The listing builds one solid part. Answer for the finished solid, in the listing's coordinates (mm). Face numbers are marked on the shaded views. A direction names the side the tool comes from. Round coordinates to 2 decimals unless told otherwise and drop trailing zeros. Write each loop counter-clockwise with the first axis right and the second up, starting at its lowest first coordinate (ties: lowest second). Pieces come first, ordered by that corner, then holes. Notation, with made-up numbers: (54.5, -29.5) - (108.5, -29.5) arc R11 cw to (108.5, -21.5) - close; hole circle Ø7 at (-7.75, 4). An arc over 180 degrees is marked (long way). Answer as CSV lines item,"result". Start each with the question number.
Item 1: Straight lines are drawn through the part: line 1 along Z through (x, y) = (9.5, 86); line 2 along Y through (x, z) = (40.5, -60.5); line 3 along Y through (x, z) = (65.5, 11). For each, find the intervals that lie inside material, in ascending order. Write a range as [from, to].
Item 2: Flat-ended cylindrical pins translate along their axes: pin 1 (4 mm diameter, centred on x = 48, y = 37, fed in from -Z); pin 2 (3 mm diameter, centred on y = -17, z = -73.5, fed in from +X); pin 3 (3 mm diameter, centred on x = 21, z = -42.5, fed in from +Y); pin 4 (6 mm diameter, centred on x = 50, y = 12.5, fed in from -Z). Find the tip coordinate at first contact, or state that the pin passes through.
Item 3: A cutting plane is placed at A-A on y = 5. Determine the outline of the cut face in (x, z).
Item 4: For a pull along Y with two mould halves and no side action, classify the marked faces 4, 5, 6 and 7 as pulls with the +Y half, pulls with the -Y half, needs draft (parallel to the pull), parting line crosses it, or undercut.
Item 5: Which of the six approach directions +Z, -Z, +X, -X, +Y, -Y give full straight-line access (tool end or side, diameter ignored) to the marked faces 1, 2 and 3?
```python
from build123d import *
from OCP.BRepFilletAPI import BRepFilletAPI_MakeChamfer

# Parameters (mm, degrees)
BOSS_EXTRUDE1_DEPTH = 90
CUT_EXTRUDE1_DEPTH  = 165.439594476
SKETCH4_R           = 37.5
CUT_EXTRUDE2_DEPTH  = 20
CUT_EXTRUDE2_DRAFT  = -6.81
SKETCH5_R           = 8
CUT_EXTRUDE3_DEPTH  = 160.138304628
SKETCH6_R           = 10
CUT_EXTRUDE4_DEPTH  = 2
FILLET1_R           = 45
CUT_EXTRUDE5_DEPTH  = 160.138304628
CHAMFER1_SIZE       = 3
CHAMFER2_SIZE       = 1
CHAMFER2_SIZE2      = 1.14368379
FILLET3_R           = 2
SKETCH8_R           = 2
CUT_EXTRUDE6_DEPTH  = 173.409396496


with BuildPart() as part:
    # Sketch1 → Boss-Extrude1 (new body)
    with BuildSketch(Plane(origin=(0, 0, 0), x_dir=(0, 0, -1), z_dir=(1, 0, 0))):
        Polygon((0, 0), (85, 0), (85, -30), (-25.553583916, -30), (-25.553583916, 100), (-9.553583916, 100), (-9.553583916, 80), align=None)
    extrude(amount=BOSS_EXTRUDE1_DEPTH)

    # Sketch2 → Cut-Extrude1 (cut, through all)
    with BuildSketch(Plane(origin=(0, 0, 9.553583916), x_dir=(-1, 0, 0), z_dir=(0, 0, -1))):
        with BuildLine():
            Line((-70.5, 95), (-70.5, 85))
            ThreePointArc((-70.5, 85), (-72.75, 82.75), (-75, 85))
            Line((-75, 85), (-75, 95))
            ThreePointArc((-75, 95), (-72.75, 97.25), (-70.5, 95))
        make_face()
        with BuildLine():
            Line((-19.5, 95), (-19.5, 85))
            ThreePointArc((-19.5, 85), (-17.25, 82.75), (-15, 85))
            Line((-15, 85), (-15, 95))
            ThreePointArc((-15, 95), (-17.25, 97.25), (-19.5, 95))
        make_face()
    extrude(amount=-CUT_EXTRUDE1_DEPTH, mode=Mode.SUBTRACT)


with BuildPart() as cut_extrude2_tool:
    # Sketch4 → Cut-Extrude2 (with draft: the straight prism first)
    with BuildSketch(Plane(origin=(0, 0, 0), x_dir=(1, 0, 0), z_dir=(0, 1, 0))):
        with Locations((45, 42.5)):
            Circle(SKETCH4_R)
    extrude(amount=-CUT_EXTRUDE2_DEPTH)
    # Cut-Extrude2: the draft: its side faces are tilted about the plane it starts from
    cut_extrude2_sides = [cut_extrude2_tool.faces().sort_by_distance(p)[0] for p in [
        (7.5, -10, -42.5),
    ]]
    draft(cut_extrude2_sides, Plane(origin=(0, 0, 0), x_dir=(1, 0, 0), z_dir=(0, 1, 0)), CUT_EXTRUDE2_DRAFT)


with BuildPart() as part_1:
    add(part.part)

    # Cut-Extrude2: cut by cut_extrude2_tool
    add(cut_extrude2_tool.part, mode=Mode.SUBTRACT)

    # Sketch5 → Cut-Extrude3 (cut, through all)
    with BuildSketch(Plane(origin=(0, 0, 0), x_dir=(-1, 0, 0), z_dir=(0, 0.11857727167698189, -0.9929448275919681))):
        with Locations(Location((-45, 55.568424123, 0), (0, 0, 90))):
            Circle(SKETCH5_R)
    extrude(amount=-CUT_EXTRUDE3_DEPTH, mode=Mode.SUBTRACT)

    # Sketch6 → Cut-Extrude4 (cut)
    with BuildSketch(Plane(origin=(0, 0, 0), x_dir=(-1, 0, 0), z_dir=(0, 0.11857727167698189, -0.9929448275919681))):
        with Locations(Location((-45, 55.568424123, 0), (0, 0, 90))):
            Circle(SKETCH6_R)
    extrude(amount=-CUT_EXTRUDE4_DEPTH, mode=Mode.SUBTRACT)

    # Fillet1
    fillet1_edges = [part_1.edges().sort_by_distance(p)[0] for p in [
        (0, -15, -85),
        (90, -15, -85),
    ]]
    fillet(fillet1_edges, radius=FILLET1_R - 0.0001)  # a hair under: the kernel refuses the full size

    # Sketch7 → Cut-Extrude5 (cut, through all)
    with BuildSketch(Plane(origin=(0, 0, 0), x_dir=(-1, 0, 0), z_dir=(0, 0.11857727167698176, -0.9929448275919681))):
        Polygon((-45, 32.853259254), (-66.213203436, 11.640055819), (-23.786796564, 11.640055819), align=None)
        Polygon((-80.494028285, 18.572434405), (-59.280824849, 39.78563784), (-80.494028285, 60.998841276), align=None)
        Polygon((-30.719175151, 39.78563784), (-9.505971715, 60.998841276), (-9.505971715, 18.572434405), align=None)
    extrude(amount=-CUT_EXTRUDE5_DEPTH, mode=Mode.SUBTRACT)

    # Chamfer1
    chamfer1_edges = [part_1.edges().sort_by_distance(p)[0] for p in [
        (34.393398282, 22.089703532, 2.637947955),
        (55.606601718, 22.089703532, 2.637947955),
        (45, 11.557933218, 1.380246061),
        (20.112573433, 28.973172992, 3.459970494),
        (9.505971715, 39.504943306, 4.717672387),
        (20.112573433, 50.03671362, 5.97537428),
        (80.494028285, 39.504943306, 4.717672387),
        (69.887426567, 28.973172992, 3.459970494),
        (69.887426567, 50.03671362, 5.97537428),
    ]]
    chamfer(chamfer1_edges, length=CHAMFER1_SIZE)

    # Chamfer2: one chamfer whose edges measure the first distance from different faces: ONE call of the kernel's chamfer builder (chamfer() names one face for all edges)
    chamfer2_edges_1 = [part_1.edges().sort_by_distance(p)[0] for p in [
        (9.888395979, -20, -42.5),
    ]]
    chamfer2_side_1 = [part_1.faces().sort_by_distance(p)[0] for p in [
        (8.694197989, -10, -42.5),
    ]]
    chamfer2_edges_2 = [part_1.edges().sort_by_distance(p)[0] for p in [
        (7.5, 0, -42.5),
    ]]
    chamfer2_side_2 = [part_1.faces().sort_by_distance(p)[0] for p in [
        (1.23794184, 0, -20.00005),
    ]]
    chamfer2 = BRepFilletAPI_MakeChamfer(part_1.part.solid().wrapped)
    for e in chamfer2_edges_1:
        chamfer2.Add(CHAMFER2_SIZE, CHAMFER2_SIZE2, e.wrapped, chamfer2_side_1[0].wrapped)  # the first distance lies on this face
    for e in chamfer2_edges_2:
        chamfer2.Add(CHAMFER2_SIZE, CHAMFER2_SIZE2, e.wrapped, chamfer2_side_2[0].wrapped)  # the first distance lies on this face
    add(Compound.cast(chamfer2.Shape()), mode=Mode.REPLACE)

    # Fillet3
    fillet3_edges = [part_1.edges().sort_by_distance(p)[0] for p in [
        (45, 11.202201403, 4.359080544),
        (55.606601718, 21.733971717, 5.616782437),
        (34.393398282, 21.733971717, 5.616782437),
        (20.112573433, 28.617441177, 6.438804976),
        (9.505971715, 39.149211491, 7.69650687),
        (20.112573433, 49.680981805, 8.954208763),
        (69.887426567, 28.617441177, 6.438804976),
        (80.494028285, 39.149211491, 7.69650687),
        (69.887426567, 49.680981805, 8.954208763),
    ]]
    fillet(fillet3_edges, radius=FILLET3_R)

    # Sketch8 → Cut-Extrude6 (cut, through all)
    with BuildSketch(Plane(origin=(0, -20, 0), x_dir=(1, 0, 0), z_dir=(0, 1, 0))):
        with Locations(Location((45, 42.5, 0), (0, 0, 270))):
            Circle(SKETCH8_R)
        with Locations(Location((45, 54.5, 0), (0, 0, 270))):
            Circle(SKETCH8_R)
        with Locations(Location((21, 42.5, 0), (0, 0, 270))):
            Circle(SKETCH8_R)
        with Locations(Location((57, 42.5, 0), (0, 0, 270))):
            Circle(SKETCH8_R)
        with Locations(Location((45, 30.5, 0), (0, 0, 270))):
            Circle(SKETCH8_R)
        with Locations(Location((33, 42.5, 0), (0, 0, 270))):
            Circle(SKETCH8_R)
        with Locations(Location((33, 63.284609691, 0), (0, 0, 270))):
            Circle(SKETCH8_R)
        with Locations(Location((57, 63.284609691, 0), (0, 0, 270))):
            Circle(SKETCH8_R)
        with Locations(Location((69, 42.5, 0), (0, 0, 270))):
            Circle(SKETCH8_R)
        with Locations(Location((57, 21.715390309, 0), (0, 0, 270))):
            Circle(SKETCH8_R)
        with Locations(Location((33, 21.715390309, 0), (0, 0, 270))):
            Circle(SKETCH8_R)
    extrude(amount=-CUT_EXTRUDE6_DEPTH, mode=Mode.SUBTRACT)


solid = part_1.part
```
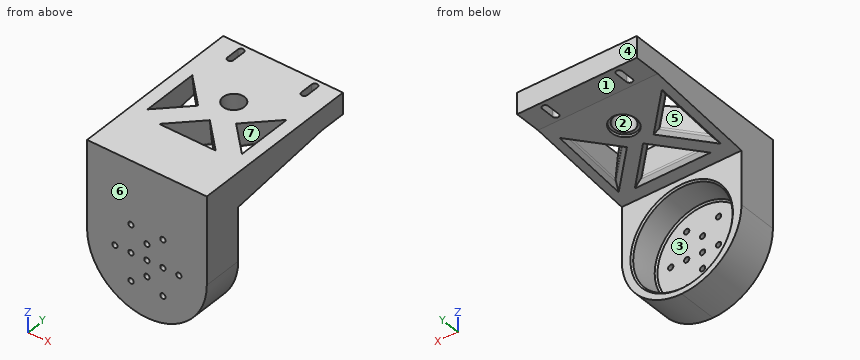
Geometry says:
1,line 1,"z = [9.55, 25.55]"
1,line 2,"y = [-30, -20]"
1,line 3,"y = [-30, 10.41], [11.13, 32.49], [45.02, 100]"
2,pin 1,"stops at z = 4.18"
2,pin 2,"stops at x = 76.64"
2,pin 3,"passes through"
2,pin 4,"stops at z = 2.2"
3,outline,"(0, 0.6) - (90, 0.6) - (90, 25.55) - (0, 25.55) - close"
4,face 4,"pulls with the +Y half"
4,face 5,"undercut"
4,face 6,"pulls with the -Y half"
4,face 7,"undercut"
5,face 1,"-Z, +X, -X, +Y"
5,face 2,"none"
5,face 3,"+Y"
